Model file for the job. Use its own axes, mm. Coordinates: 2 decimals unless noted, no trailing zeros. Write each loop counter-clockwise with the first axis right and the second up, starting at its lowest first coordinate (ties: lowest second). Pieces come first, ordered by that corner, then holes. Notation, with made-up numbers: M -13.75,-13.75 L 21.25,-13.75 A25 cw 21.25,10.25 Z; hole C 29,87 d2. An arc over 180 degrees is marked long. Put each result on its own line as item: value. Start each with the question number.
Q1. Drill centre lines: line 1 along X through (y, z) = (130, 0.95) (3 decimals); line 2 along X through (y, z) = (250, 0.75); line 3 along Y through (x, z) = (10, 1.4) (3 decimals). Where is each one in solid material? Low to high.
Q2. Cut at A-A (x = 78.5). Write the cut outline in (y, z).
Q3. Cut at B-B (y = 194.5). Write the cut outline in (x, z).
Q4. Cut at C-C (z = 1.1). Write the cut outline in (x, y) (3 decimals), then the cut area to 3 significant figures.
```python
from build123d import *

# Parameters (mm, degrees)
SKETCH_1_W          = 130
SKETCH_1_H          = 260
EXTRUDE_1_DEPTH     = 3
SKETCH_2_R          = 1.65
SKETCH_2_R_2        = 1.6
SKETCH_2_R_3        = 1.605
CUT_EXTRUDE_1_DEPTH = 3
SKETCH_3_W          = 50
SKETCH_3_H          = 50
CUT_EXTRUDE_2_DEPTH = 10
FILLET_1_R          = 15


with BuildPart() as part:
    # 草图1 → 凸台-拉伸1 (new body)
    with BuildSketch(Plane.XY):
        with Locations((65, 130)):
            Rectangle(SKETCH_1_W, SKETCH_1_H)
    extrude(amount=EXTRUDE_1_DEPTH)

    # 草图2 → 切除-拉伸1 (cut)
    with BuildSketch(Plane.XY.offset(3)):
        with Locations((120, 10)):
            Circle(SKETCH_2_R)
        with Locations((10, 10)):
            Circle(SKETCH_2_R)
        with Locations(Location((10, 250, 0), (0, 0, 180))):
            Circle(SKETCH_2_R)
        with Locations(Location((120, 250, 0), (0, 0, 180))):
            Circle(SKETCH_2_R)
        with Locations((120, 130)):
            Circle(SKETCH_2_R_2)
        with Locations((10, 130)):
            Circle(SKETCH_2_R_3)
    extrude(amount=-CUT_EXTRUDE_1_DEPTH, mode=Mode.SUBTRACT)

    # 草图3 → 切除-拉伸2 (cut)
    with BuildSketch(Plane(origin=(0, 0, 0), x_dir=(-1, 0, 0), z_dir=(0, 0, -1))):
        with Locations((-65, 180)):
            Rectangle(SKETCH_3_W, SKETCH_3_H)
    extrude(amount=-CUT_EXTRUDE_2_DEPTH, mode=Mode.SUBTRACT)

    # 圆角1
    fillet_1_edges = [part.edges().sort_by_distance(p)[0] for p in [
        (0, 0, 1.5),
        (130, 0, 1.5),
        (130, 260, 1.5),
        (0, 260, 1.5),
    ]]
    fillet(fillet_1_edges, radius=FILLET_1_R)


solid = part.part
```
Computed values:
1. line 1: 0 to 8.395, 11.605 to 118.4, 121.6 to 130
1. line 2: 0.86 to 8.35, 11.65 to 118.35, 121.65 to 129.14
1. line 3: 0.858 to 8.35, 11.65 to 128.395, 131.605 to 248.35, 251.65 to 259.142
2. outline: M 0,0 L 155,0 L 155,3 L 0,3 Z; M 205,0 L 260,0 L 260,3 L 205,3 Z
3. outline: M 0,0 L 40,0 L 40,3 L 0,3 Z; M 90,0 L 130,0 L 130,3 L 90,3 Z
4. outline: M 0,15 A15 ccw 15,0 L 115,0 A15 ccw 130,15 L 130,245 A15 ccw 115,260 L 15,260 A15 ccw 0,245 Z; hole C 10,10 d3.3; hole C 10,250 d3.3; hole C 10,130 d3.21; hole M 40,155 L 90,155 L 90,205 L 40,205 Z; hole C 120,10 d3.3; hole C 120,250 d3.3; hole C 120,130 d3.2
4. area: 31,100 mm2
